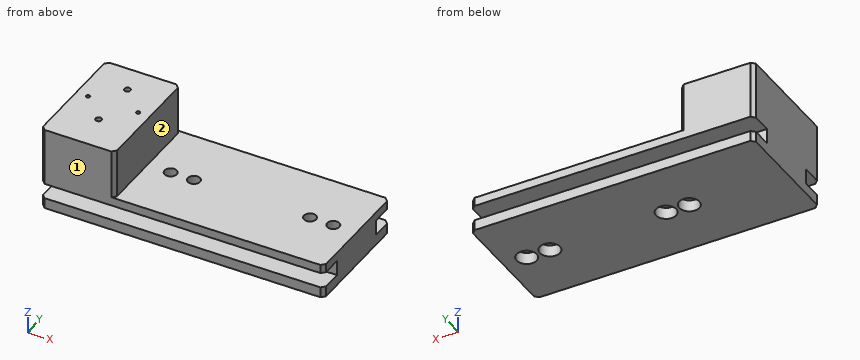
Autodesk Inventor part; units mm, degrees
ref_plane "YZ Plane" through (0, 0, 0) normal (1, 0, 0) x (0, 1, 0)
ref_plane "XZ Plane" through (0, 0, 0) normal (0, 1, 0) x (-1, 0, 0)
ref_plane "XY Plane" through (0, 0, 0) normal (0, 0, 1) x (1, 0, 0)
sketch "Sketch1" plane through (0, 0, 0) normal (0, 0, 1) x (1, 0, 0)
  line L0 (-40.45, 31.75) -> (114.3, 31.75)
  line L1 (114.3, 31.75) -> (114.3, -31.75)
  line L2 (114.3, -31.75) -> (-40.45, -31.75)
  line L3 (-40.45, -31.75) -> (-40.45, 31.75)
  point P0 (0, 0)
  dimension "d0" = 63.5
  dimension "d1" = 31.75
  dimension "d2" = 40.45
  dimension "LENGTH" = 154.75
extrude "Extrusion1" add sketch "Sketch1" along normal blind 18.9
sketch "Sketch2" plane through (0, 0, 18.9) normal (0, 0, 1) x (1, 0, 0)
  line L0 (114.3, 31.75) -> (-40.45, 31.75)
  line L1 (-40.45, -31.75) -> (114.3, -31.75)
  line L2 (-40.45, 31.75) -> (0, 31.75)
  line L3 (0, 31.75) -> (0, -31.75)
  line L4 (0, -31.75) -> (-40.45, -31.75)
  line L5 (-40.45, -31.75) -> (-40.45, 31.75)
  point P0 (0, 0)
  dimension "d6" = 40.45
extrude "Extrusion2" add sketch "Sketch2" along normal blind 26.759
sketch "Sketch3" plane through (0, 0, 0) normal (0, 0, 1) x (1, 0, 0)
  line L0 (114.3, -31.75) -> (114.3, 31.75)
  point P0 (0, 0)
  point P1 (12.7, 0)
  point P2 (25.4, 0)
  point P3 (88.9, 0)
  point P4 (101.6, 0)
  dimension "d9" = 0
  dimension "d10" = 0
  dimension "d11" = 0
  dimension "d12" = 0
  dimension "d13" = 88.9
  dimension "d14" = 12.7
  dimension "d15" = 63.5
  dimension "d16" = 12.7
hole "Hole2" at (12.7, 0, 0) at (101.6, 0, 0) at (25.4, 0, 0) at (88.9, 0, 0) direction (0, 0, 1) diameter 6.7 end through all counterbore diameter 11 counterbore depth 6.4
sketch "Sketch4" plane through (-40.45, -31.75, 0) normal (0, -1, 0) x (1, 0, 0)
  line L0 (0, 5.775) -> (154.75, 5.775)
  line L1 (154.75, 5.775) -> (154.75, 14.125)
  line L2 (154.75, 14.125) -> (0, 14.125)
  line L3 (0, 14.125) -> (0, 5.775)
  line L4 (0, 5.775) -> (154.75, 14.125) construction
  line L5 (154.75, 5.775) -> (0, 14.125) construction
  line L6 (0, 0) -> (0, 45.659)
  line L7 (0, 0) -> (154.75, 0)
  point P0 (40.45, 0)
  point P1 (77.375, 9.95)
  dimension "d31" = 154.75
  dimension "d32" = 77.375
  dimension "d33" = 9.95
  dimension "SLOT_HEIGHT" = 8.35
sketch "Sketch5" plane through (-40.45, 31.75, 0) normal (0, 1, 0) x (1, 0, 0)
  line L0 (154.75, -5.775) -> (0, -5.775)
  line L1 (0, -5.775) -> (0, -14.125)
  line L2 (0, -14.125) -> (154.75, -14.125)
  line L3 (154.75, -14.125) -> (154.75, -5.775)
  line L4 (154.75, -5.775) -> (0, -14.125) construction
  line L5 (0, -5.775) -> (154.75, -14.125) construction
  line L6 (0, 0) -> (0, -45.659)
  point P0 (40.45, 0)
  point P1 (77.375, -9.95)
  dimension "d35" = 8.35
  dimension "d36" = 154.75
  dimension "d37" = 0
  dimension "d38" = 9.95
extrude "Extrusion3" cut sketch "Sketch5" against normal blind 12.7
extrude "Extrusion4" cut sketch "Sketch4" against normal blind 12.7
sketch "Sketch6" plane through (0, 0, 45.659) normal (0, 0, 1) x (1, 0, 0)
  line L0 (0, 31.75) -> (-40.45, 31.75)
  line L1 (-40.45, -31.75) -> (0, -31.75)
  line L2 (-40.45, 31.75) -> (-40.45, -31.75)
  line L3 (-6.575, 2.048) -> (-6.575, 3.048) construction
  line L4 (-5.525, 2.048) -> (-5.525, 3.048)
  line L5 (-7.625, 3.048) -> (-7.625, 2.048)
  arc A0 (-7.625, 2.048) -> (-5.525, 2.048) centre (-6.575, 2.048) ccw
  arc A1 (-5.525, 3.048) -> (-7.625, 3.048) centre (-6.575, 3.048) ccw
  point P0 (0, 0)
  point P1 (-20.225, -11.502)
  point P2 (-20.225, 16.598)
  point P3 (-33.875, 2.548)
  point P4 (-6.575, 2.548)
  dimension "d43" = 0
  dimension "d44" = 15.152
  dimension "d45" = 0
  dimension "d46" = 20.248
  dimension "d47" = 20.225
  dimension "d48" = 28.1
  dimension "d50" = 27.3
  dimension "d51" = 14.05
  dimension "d52" = 13.65
  dimension "d67" = 1.05
  dimension "d68" = 1
hole "Hole3" at (-33.875, 2.548, 45.659) at (-6.575, 2.548, 45.659) direction (0, 0, -1) diameter 2.1 depth 4.1
hole "Hole4" at (-20.225, -11.502, 45.659) at (-20.225, 16.598, 45.659) direction (0, 0, -1) diameter 3.302 depth 12.3
chamfer "Chamfer1" [suppressed]
chamfer "Chamfer2" distance 2 angle 45 10 edges at (0, -31.75, 32.2795) (-40.45, -31.75, 29.892) (-40.45, -31.75, 2.8875) (114.3, -31.75, 16.5125) (114.3, -31.75, 2.8875) (114.3, 31.75, 16.5125) (114.3, 31.75, 2.8875) (0, 31.75, 32.2795) (-40.45, 31.75, 29.892) (-40.45, 31.75, 2.8875)
equation "\"d0\" = WIDTH"
equation "\"LENGTH\" = APP_LENGTH + ISOLATOR_MT_LENGTH"
equation "\"d6\" = APP_LENGTH"
equation "\"d7\" = APP_HEIGHT"
equation "\"d31\" = LENGTH"
equation "\"d35\" = SLOT_HEIGHT"
equation "\"d36\" = LENGTH"
equation "\"d41\" = SLOT_DEPTH"
equation "\"ISOLATOR_MT_LENGTH\" = 114.3"
equation "\"WIDTH\" = 63.5"
equation "\"ISOLATOR_HEIGHT\" = 19.9"
equation "\"APP_LENGTH\" = 40.45"
equation "\"APP_HEIGHT\" = 26.759"
properties part number "711C-1-APP-mount"
Input: part model. Units: mm. Frame: model coordinates. Face numbers are marked on the shaded views. A direction names the side the tool comes from. Coordinates: 2 decimals unless noted, no trailing zeros. Write each loop counter-clockwise with the first axis right and the second up, starting at its lowest first coordinate (ties: lowest second). Pieces come first, ordered by that corner, then holes. Notation, with made-up numbers: (43, -0.75) - (69, -0.75) arc R4 ccw to (69, 4.25) - close; hole circle Ø3 at (-6, 60.5). An arc over 180 degrees is marked (long way). Put each result on its own line as item: value. Start each with the question number.
1) Reachability of the marked faces 1 and 2 from +Z, -Z, +X, -X, +Y, -Y: full face, straight path, thin tool, end or side. Return the list, or none.
2) Cut plane B-B (z = 10.5). Return the cut outline in (x, y).
3) Ray query, L1, parallel to X at y = 0, z = 16.25; L2, parallel to Z at x = 76, y = -20 (3 decimals); L3, parallel to X at y = 0, z = 3. Return the intervals inside material, ascending.
4) Contact query for flat-ended pins moving along their axis: pin 1 (2 mm diameter, centred on x = 49.5, y = -5.5, fed in from +Z); pin 2 (12 mm diameter, centred on x = 68, z = 25, fed in from -Y); pin 3 (1.5 mm diameter, centred on y = 12.5, z = 30.5, fed in from +X); pin 4 (8.5 mm diameter, centred on x = 88.9, y = 0, fed in from -Z). Output: stop coordinate, or through.
5) Cut plane C-C (x = 25.4). Return the cut outline in (y, z) (3 decimals), plus the area to 3 significant figures.
6) Cut plane A-A (y = -25). Return the cut outline in (x, z) (3 decimals).
7) Cut plane D-D (z = 25). Return the cut outline in (x, y).
Resolved:
1. face 1: +Z, -Z, +X, -X, -Y
1. face 2: +Z, +X, +Y, -Y
2. outline: (-40.45, -19.05) - (114.3, -19.05) - (114.3, 19.05) - (-40.45, 19.05) - close; hole circle Ø6.7 at (12.7, 0); hole circle Ø6.7 at (25.4, 0); hole circle Ø6.7 at (88.9, 0); hole circle Ø6.7 at (101.6, 0)
3. L1: x = -40.45 to 9.35, 16.05 to 22.05, 28.75 to 85.55, 92.25 to 98.25, 104.95 to 114.3
3. L2: z = 0 to 5.775, 14.125 to 18.9
3. L3: x = -40.45 to 7.2, 18.2 to 19.9, 30.9 to 83.4, 94.4 to 96.1, 107.1 to 114.3
4. pin 1: stops at z = 18.9
4. pin 2: passes through
4. pin 3: stops at x = 0
4. pin 4: stops at z = 6.4
5. outline: (-31.75, 0) - (-5.5, 0) - (-5.5, 6.4) - (-3.35, 6.4) - (-3.35, 18.9) - (-31.75, 18.9) - (-31.75, 14.125) - (-19.05, 14.125) - (-19.05, 5.775) - (-31.75, 5.775) - close; (3.35, 6.4) - (5.5, 6.4) - (5.5, 0) - (31.75, 0) - (31.75, 5.775) - (19.05, 5.775) - (19.05, 14.125) - (31.75, 14.125) - (31.75, 18.9) - (3.35, 18.9) - close
5. area: 834 mm2
6. outline: (-40.45, 0) - (114.3, 0) - (114.3, 5.775) - (-40.45, 5.775) - close; (-40.45, 14.125) - (114.3, 14.125) - (114.3, 18.9) - (0, 18.9) - (0, 45.659) - (-40.45, 45.659) - close
7. outline: (-40.45, -29.75) - (-38.45, -31.75) - (-2, -31.75) - (0, -29.75) - (0, 29.75) - (-2, 31.75) - (-38.45, 31.75) - (-40.45, 29.75) - close
